from build123d import *

# Parameters (mm, degrees)
BOSS_EXTRUDE1_DEPTH              = 3.175
SKETCH2_R                        = 3.302
CUT_EXTRUDE1_DEPTH               = 3.175
SKETCH3_R                        = 3.302
CUT_EXTRUDE2_DEPTH               = 3.175
F_25_64_0_39063_DIAMETER_HOLE1_D = 9.922002


with BuildPart() as part:
    # Sketch1 → Boss-Extrude1 (new body)
    with BuildSketch(Plane.XY):
        with BuildLine():
            Line((-150.65739054, -36.5125), (-189.445196846, -36.5125))
            ThreePointArc((-189.445196846, -36.5125), (-175.12424315, 73.983329), (-101.363819659, 157.492716901))
            ThreePointArc((-101.363819659, 157.492716901), (-68.153294369, 173.730017516), (-32.46878203, 183.38426531))
            Line((-32.46878203, 183.38426531), (-81.449197888, 125.011678745))
            ThreePointArc((-81.449197888, 125.011678745), (-141.744884659, 55.257653644), (-150.65739054, -36.5125))
        make_face()
    extrude(amount=BOSS_EXTRUDE1_DEPTH)

    # Sketch2 → Cut-Extrude1 (cut)
    with BuildSketch(Plane.XY.offset(3.175)):
        with Locations((-166.205357894, -15.073647178)):
            Circle(SKETCH2_R)
        with Locations((-164.125827505, 29.433503815)):
            Circle(SKETCH2_R)
    extrude(amount=-CUT_EXTRUDE1_DEPTH, mode=Mode.SUBTRACT)

    # Sketch3 → Cut-Extrude2 (cut)
    with BuildSketch(Plane.XY.offset(3.175)):
        with Locations((-173.718655592, 7.579557452)):
            Circle(SKETCH3_R)
        with Locations((-166.564839951, 51.569288407)):
            Circle(SKETCH3_R)
    extrude(amount=-CUT_EXTRUDE2_DEPTH, mode=Mode.SUBTRACT)

    # 25/64 (0.39063) Diameter Hole1 (through all)
    with Locations(Plane.XY.offset(3.175)):
        with Locations((-94.36092612, 138.93426531), (-152.733512685, 89.953849452)):
            Hole(F_25_64_0_39063_DIAMETER_HOLE1_D / 2)


solid = part.part
Verification items for the finished model (mm, model axes). Round coordinates to 2 decimals unless told otherwise and drop trailing zeros. Loops run counter-clockwise (first coordinate to the right, second up) from the corner with the lowest first, then second, coordinate; pieces in that order, holes last. Notation, with made-up numbers: (18, -0.75) - (41, -0.75) arc R22 cw to (41, 35.25) - close; hole circle Ø7 at (81.25, 56.25). An arc over 180 degrees is marked (long way). Use one line per item in the form item = value.
1. Draft check along Y on faces 1 (the flat face through (-136, 74, 3.175)), 2 (the cylindrical face through (-169.864, 51.714, 1.61)), 3 (the cylindrical face through (-175.773, 72.539, 1.565)), 4 (the cylindrical face through (-97.028, 143.117, 1.565)). Enter one of: pulls with the +Y half, pulls with the -Y half, needs draft (parallel to the pull), parting line crosses it, or undercut.
A:
face_1 = needs draft
face_2 = undercut
face_3 = parting line crosses it
face_4 = undercut
2. Section check D-D on x = -112. Record the cut outline in (y, z) (3 decimals), and give its area (3 significant figures).
A:
outline = (100.332, 0) - (150.471, 0) - (150.471, 3.175) - (100.332, 3.175) - close
area = 159 mm²
3. Section check B-B on z = 2.25. Record the cut outline in (x, y).
A:
outline = (-189.45, -36.51) - (-150.66, -36.51) arc R152.08 cw to (-81.45, 125.01) - (-32.47, 183.38) arc R194.32 ccw to (-101.36, 157.49) arc R190.18 ccw to start; hole circle Ø6.6 at (-173.72, 7.58); hole circle Ø6.6 at (-166.56, 51.57); hole circle Ø6.6 at (-166.21, -15.07); hole circle Ø6.6 at (-164.13, 29.43); hole circle Ø9.92 at (-152.73, 89.95); hole circle Ø9.92 at (-94.36, 138.93)
4. Section check A-A on x = -95.5. Record the cut outline in (y, z) (1 decimal).
A:
outline = (115.3, 0) - (134.1, 0) - (134.1, 3.2) - (115.3, 3.2) - close; (143.8, 0) - (160.9, 0) - (160.9, 3.2) - (143.8, 3.2) - close
5. Scan lines: probe 1 along Y at (x, z) = (-168.5, 2.6); probe 2 along X at (y, z) = (86, 1); probe 3 along X at (y, z) = (135, 0.6). Record each from-to range of solid material in increasing order.
A:
probe_1 = -36.51 to -17.45, -12.7 to 48.89, 54.24 to 87.19
probe_2 = -169.15 to -155.73, -149.74 to -124.08
probe_3 = -131.07 to -97.38, -91.34 to -73.07
6. Section check C-C on y = 76.5. Record the cut outline in (x, z) (3 decimals), and give its area (3 significant figures).
A:
outline = (-173.959, 0) - (-130.584, 0) - (-130.584, 3.175) - (-173.959, 3.175) - close
area = 138 mm²
7. Gauge pin test, flat ends, axial feed: pin 1 Ø13 at (x, y) = (-152.73, 89.95) entering from +Z (3 decimals); pin 2 Ø5.5 at (x, y) = (-166.21, -15.07) entering from -Z; pin 3 Ø1.5 at (y, z) = (137, 1) entering from -X; pin 4 Ø1 at (y, z) = (107, 1) entering from +X. Record the tip position at first contact, or that the pin passes through.
A:
pin_1 = 3.175
pin_2 = through
pin_3 = -129.7
pin_4 = -104.69
